Read the model definition and answer for the solid it produces. Units are mm, in the model's axes. A direction names the side the tool comes from. Coordinates: 2 decimals unless noted, no trailing zeros. Loops run counter-clockwise (first coordinate to the right, second up) from the corner with the lowest first, then second, coordinate; pieces in that order, holes last. Notation, with made-up numbers: M 16,78 L 63,78 A28 ccw 63,112 Z; hole C 43,56.25 d7. An arc over 180 degrees is marked long. Put each result on its own line as item: value.
Autodesk Inventor part; units mm, degrees
ref_plane "YZ Plane" through (0, 0, 0) normal (1, 0, 0) x (0, 1, 0)
ref_plane "XZ Plane" through (0, 0, 0) normal (0, 1, 0) x (-1, 0, 0)
ref_plane "XY Plane" through (0, 0, 0) normal (0, 0, 1) x (1, 0, 0)
sketch "Sketch6" plane through (0, 0, 0) normal (0, 0, 1) x (1, 0, 0)
  arc A0 (9, 95.047) -> (2, 95.047) centre (5.5, 99.2896) ccw
  arc A1 (2, 9.7426) -> (9, 9.7426) centre (5.5, 5.5) ccw
  circle A2 centre (5.5, 5.5) radius 3.5
  circle A3 centre (5.5, 99.2896) radius 3.5
  line L0 (2, 95.047) -> (2, 9.7426)
  line L1 (9, 9.7426) -> (9, 95.047)
  point P0 (0, 0)
  dimension "d89" = 93.7896
  dimension "d90" = 7
  dimension "d91" = 7
  dimension "d92" = 5.5
  dimension "d93" = 7
  dimension "d94" = 5.5
extrude "Extrusion3" add sketch "Sketch6" along normal blind 3
properties part number "4P.01.02.28-BC-v1-Final Aileron L3 80deg" material "Acrylic, Clear"
1) Find section D-D, the plane y = 34. Write down the section's boundary in (x, z).
Answer list:
outline: M 2,0 L 9,0 L 9,3 L 2,3 Z
2) Find section C-C, the plane z = 0.9. Write down the section's boundary in (x, y), plus the area to 3 significant figures.
Answer list:
outline: M 2,9.74 A5.5 ccw long 9,9.74 L 9,95.05 A5.5 ccw long 2,95.05 Z; hole C 5.5,5.5 d7; hole C 5.5,99.29 d7
area: 698 mm^2
3) Straight lines are drawn through the part: line 1 (Y direction, x = 5.25, z = 2.5); line 2 (Y direction, x = 1.25, z = 1); line 3 (Y direction, x = 2.5, z = 0.4). For each, find the intervals that lie inside material, in ascending order. Write a range as [from, to].
Answer list:
line 1: y = [0.01, 2.01], [8.99, 95.8], [102.78, 104.78]
line 2: y = [2.01, 8.99], [95.8, 102.78]
line 3: y = [0.89, 3.7], [7.3, 97.49], [101.09, 103.9]
4) Determine the mould class of faces 3 (the flat face through (5, 53, 3)), 4 (the flat face through (9, 52, 1)) for opening direction Y: released by +Y, released by -Y, zero draft, split by the parting line, or undercut.
Answer list:
face 3: zero draft
face 4: undercut
5) Find section B-B, the plane x = 5.5. Write down the section's boundary in (y, z), plus the area to 3 significant figures.
Answer list:
outline: M 0,0 L 2,0 L 2,3 L 0,3 Z; M 9,0 L 95.79,0 L 95.79,3 L 9,3 Z; M 102.79,0 L 104.79,0 L 104.79,3 L 102.79,3 Z
area: 272 mm^2
6) Find section A-A, the plane y = 5.5. Write down the section's boundary in (x, z).
Answer list:
outline: M 0,0 L 2,0 L 2,3 L 0,3 Z; M 9,0 L 11,0 L 11,3 L 9,3 Z
7) Which of the six approach directions +Z, -Z, +X, -X, +Y, -Y give full straight-line access (tool end or side, diameter ignored) to faces 1 (the cylindrical face through (5.689, 0.003, 1.479)), 2 (the flat face through (2, 53, 1))?
Answer list:
face 1: +Z, -Z
face 2: +Z, -Z, -X
8) Given pin 1 Ø6 at (x, y) = (10, 90) entering from -Z, flat-ended and moving along its own axis, determine where the tip first touches the part or whether it passes through.
Answer list:
pin 1: stops at z = 0
